The listing builds one solid part. Answer for the finished solid, in the listing's coordinates (mm). A direction names the side the tool comes from. Give positions to 0.01 mm unless a question says otherwise; leave off trailing zeros. Order: outer loops, then holes, each group sorted by start corner. A loop starts at its lowest first (then second) coordinate and runs counter-clockwise, first axis right, second up. Notation, with made-up numbers: (21, -33.75) - (41, -33.75) arc R13 cw to (41, -26.75) - close; hole circle Ø7 at (68, 45). An arc over 180 degrees is marked (long way). Answer in a Markdown table with one row per item.
Autodesk Inventor part; units mm, degrees
ref_plane "Start Plane" through (0, 0, 50) normal (0, 0, 1) x (1, 0, 0)
ref_plane "End Plane" through (0, 0, 525) normal (0, 0, 1) x (1, 0, 0)
ref_plane "Work Plane4" through (42.5, -515, 50) normal (0, 0, -1) x (-1, 0, 0)
ref_plane "Start Plane" through (0, 0, 50) normal (0, 0, 1) x (1, 0, 0)
ref_plane "End Plane" through (0, 0, 525) normal (0, 0, 1) x (1, 0, 0)
sketch "Sketch" plane through (0, 0, 0) normal (0, 0, 1) x (1, 0, 0)
  line L0 (-50, -42.5) -> (-50, 42.5)
  line L1 (-42.5, 50) -> (42.5, 50)
  line L2 (50, 42.5) -> (50, -42.5)
  line L3 (42.5, -50) -> (-42.5, -50)
  arc A0 (-50, -42.5) -> (-42.5, -50) centre (-42.5, -42.5) ccw
  arc A1 (-42.5, 50) -> (-50, 42.5) centre (-42.5, 42.5) ccw
  arc A2 (50, 42.5) -> (42.5, 50) centre (42.5, 42.5) ccw
  arc A3 (42.5, -50) -> (50, -42.5) centre (42.5, -42.5) ccw
  line L4 (-40, 45) -> (40, 45)
  line L5 (45, 40) -> (45, -40)
  line L6 (40, -45) -> (-40, -45)
  line L7 (-45, -40) -> (-45, 40)
  line L8 (0, 72.1746) -> (0, -72.1746) construction
  line L9 (-72.1746, 0) -> (72.1746, 0) construction
  arc A4 (-45, -40) -> (-40, -45) centre (-40, -40) ccw
  arc A5 (-40, 45) -> (-45, 40) centre (-40, 40) ccw
  arc A6 (45, 40) -> (40, 45) centre (40, 40) ccw
  arc A7 (40, -45) -> (45, -40) centre (40, -40) ccw
  dimension "d7" = 7.5
  dimension "d10" = 100
  dimension "d11" = 100
  dimension "d12" = 5
  dimension "d15" = 50
  dimension "d16" = 50
  dimension "d19" = 5
  dimension "d20" = 5
extrude "Body" add sketch "Sketch" along normal up to surface (475 mm away) from surface at 50
sketch "Sketch3" plane through (0, 0, 0) normal (0, 0, 1) x (1, 0, 0)
  line L0 (0, 0) -> (10, 0)
ref_plane "Work Plane3" through (0, 0, 0) normal (0, -1, 0) x (1, 0, 0)
ref_plane "Work Plane4" through (42.5, -515, 50) normal (0, 0, -1) x (-1, 0, 0)
split "Split1" plane through (42.5, -515, 50) removes the side toward (0, 0, -1)
sketch "Sketch4" plane through (0, 0, 0) normal (0, -1, 0) x (1, 0, 0)
  line L0 (-2, 50) -> (12, 50)
  line L1 (-2, 525) -> (12, 525)
  dimension "d18" = 475
equation "\"d7\" = G_IR"
equation "\"d10\" = G_H"
equation "\"d11\" = G_W"
equation "\"d12\" = G_T"
equation "\"d15\" = 0.5 * d10"
equation "\"d16\" = 0.5 * d11"
equation "\"d19\" = G_T"
equation "\"d20\" = G_T"
equation "\"d3\" = G_L"
equation "\"G_W\" = 100"
equation "\"G_H\" = 100"
equation "\"G_T\" = 5"
equation "\"G_IR\" = 7.5"
equation "\"G_L\" = d18"
equation "\"G_OFFSET_END\" = 0"
equation "\"d14\" = G_OFFSET_END + B_L"
equation "\"B_L\" = 525"
properties part number "DIN EN 10210-2 - 100 x 100 x 5 - 475" material "Steel, Mild"
Item 1: Which of the six approach directions +Z, -Z, +X, -X, +Y, -Y give full straight-line access (tool end or side, diameter ignored) to faces 5 (the face through (45, 1, 284)), 6 (the face through (47.745, 47.861, 284.175))?
Answer block:
| item | result |
|---|---|
| face 5 | +Z, -Z |
| face 6 | +Z, -Z, +X, +Y |
Item 2: Find section C-C on z = 159. Write down the section's boundary in (x, y), then the cut area to 3 significant figures.
Answer block:
| item | result |
|---|---|
| outline | (-50, -42.5) arc R7.5 ccw to (-42.5, -50) - (42.5, -50) arc R7.5 ccw to (50, -42.5) - (50, 42.5) arc R7.5 ccw to (42.5, 50) - (-42.5, 50) arc R7.5 ccw to (-50, 42.5) - close; hole (-45, -40) arc R5 ccw to (-40, -45) - (40, -45) arc R5 ccw to (45, -40) - (45, 40) arc R5 ccw to (40, 45) - (-40, 45) arc R5 ccw to (-45, 40) - close |
| area | 1,870 mm² |
Item 3: Consider line 1 (Y direction, x = -30, z = 221); line 2 (Y direction, x = -43, z = 465.5). Determine where each line is inside the solid, lowest interval first.
Answer block:
| item | result |
|---|---|
| line 1 | -50 to -45, 45 to 50 |
| line 2 | -49.98 to -44, 44 to 49.98 |
Item 4: Find section A-A on x = 29. Write down the section's boundary in (y, z), then the cut area to 3 significant figures.
Answer block:
| item | result |
|---|---|
| outline | (-50, 50) - (-45, 50) - (-45, 525) - (-50, 525) - close; (45, 50) - (50, 50) - (50, 525) - (45, 525) - close |
| area | 4,750 mm² |
Item 5: Determine the mould class of faces 1 (the face through (-1, 45, 284)), 2 (the face through (47.861, -47.745, 284.175)), 3 (the face through (-45, -1, 284)), 4 (the face through (1, -50, 284)) for opening direction X: pulls with the +X half, pulls with the -X half, needs draft (parallel to the pull), parting line crosses it, or undercut.
Answer block:
| item | result |
|---|---|
| face 1 | undercut |
| face 2 | pulls with the +X half |
| face 3 | undercut |
| face 4 | needs draft |
